Drawing for the job (mm, zero at the part's lowest x, y, z). Coordinates: 2 decimals unless noted, no trailing zeros. Write each loop counter-clockwise with the first axis right and the second up, starting at its lowest first coordinate (ties: lowest second). Pieces come first, ordered by that corner, then holes. Notation, with made-up numbers: M 59.5,44 L 102.5,44 A30 ccw 102.5,75 Z; hole C -23.5,77.25 d7. An arc over 180 degrees is marked long. Put each result on its own line as item: value. Start each with the question number.
Q1. Cut at A-A (z = 75). Write the cut outline in (x, y), then the cut area to 3 significant figures.
Q2. Drop flat-ended pins along their axis: pin 1 (6 mm diameter, centred on x = 108.5, z = 20.5, fed in from +Y); pin 2 (1 mm diameter, centred on y = 9.5, z = 30, fed in from -X); pin 3 (2 mm diameter, centred on y = 12, z = 56.5, fed in from +X). Give the stop position or say it passes through.
Q3. Cut at B-B (y = 27.5). Write the cut outline in (x, z) (1 decimal), then the cut area to 3 significant figures.
Q4. Drill centre lines: line 1 along Y through (x, z) = (51.5, 34); line 2 along X through (y, z) = (12, 72); line 3 along X through (y, z) = (30, 61.5). Where is each one in solid material? Low to high.
Q5. Cut at C-C (x = 31.5). Write the cut outline in (y, z).
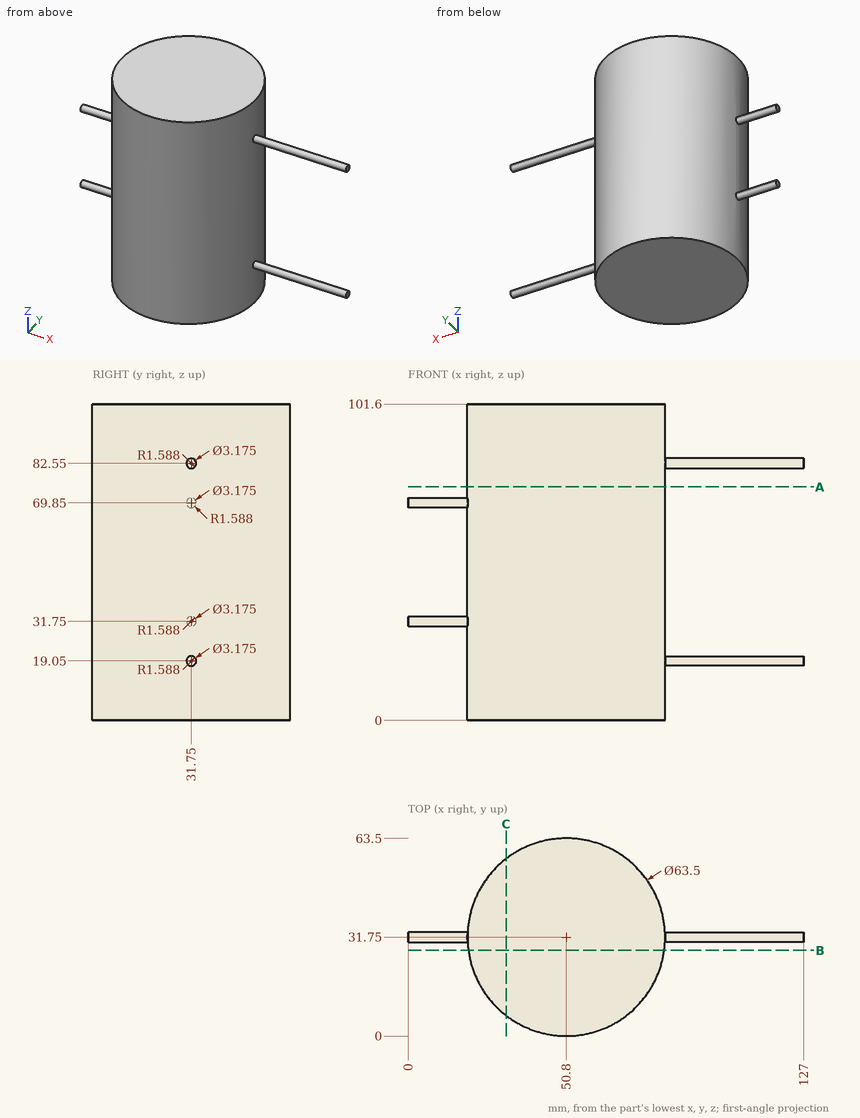
Computed values:
1. outline: C 50.8,31.75 d63.5
1. area: 3,170 mm2
2. pin 1: y = 33.34
2. pin 2: x = 27.67
2. pin 3: x = 76.42
3. outline: M 19.3,0 L 82.3,0 L 82.3,101.6 L 19.3,101.6 Z
3. area: 6,390 mm2
4. line 1: 0.01 to 63.49
4. line 2: 25.94 to 75.66
4. line 3: 19.1 to 82.5
5. outline: M 6.54,0 L 56.96,0 L 56.96,101.6 L 6.54,101.6 Z
